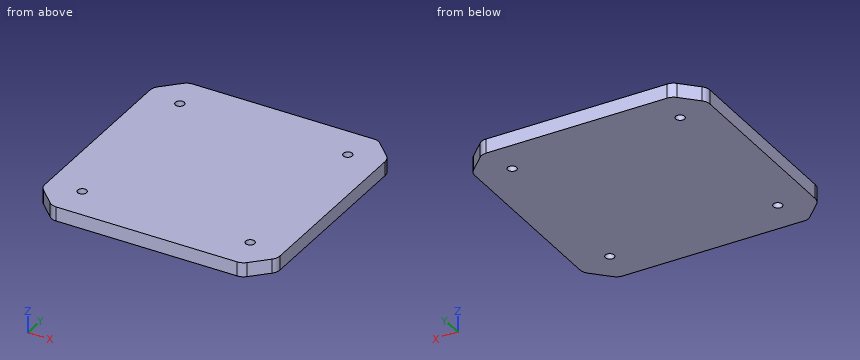
from build123d import *

# Parameters (mm, degrees)
F0_W     = 105
F0_H     = 105
F0_R     = 2
F1_DEPTH = 6.35
F2_SIZE  = 10
F3_R     = 5


# Not quite as in the source:
# - a length typed as a fraction of an inch, garbled in the dataset ("3 / 203.2 mm" for 3/8 in), is restored


with BuildPart() as f1:
    # F0 (on Top) → F1 (new body)
    with BuildSketch(Plane.XY):
        Rectangle(F0_W, F0_H)
        with Locations((-37.5, -37.5)):
            Circle(F0_R, mode=Mode.SUBTRACT)
        with Locations((37.5, -37.5)):
            Circle(F0_R, mode=Mode.SUBTRACT)
        with Locations((-37.5, 37.5)):
            Circle(F0_R, mode=Mode.SUBTRACT)
        with Locations((37.5, 37.5)):
            Circle(F0_R, mode=Mode.SUBTRACT)
    extrude(amount=F1_DEPTH)

    # F2
    f2_edges = [f1.edges().sort_by_distance(p)[0] for p in [
        (-52.5, -52.5, 3.175),
        (52.5, -52.5, 3.175),
        (52.5, 52.5, 3.175),
        (-52.5, 52.5, 3.175),
    ]]
    chamfer(f2_edges, length=F2_SIZE)

    # F3
    f3_edges = [f1.edges().sort_by_distance(p)[0] for p in [
        (52.5, 42.5, 3.175),
        (42.5, 52.5, 3.175),
        (-42.5, 52.5, 3.175),
        (-52.5, 42.5, 3.175),
        (-52.5, -42.5, 3.175),
        (-42.5, -52.5, 3.175),
        (42.5, -52.5, 3.175),
        (52.5, -42.5, 3.175),
    ]]
    fillet(f3_edges, radius=F3_R)


solid = f1.part
Input: part model. Units: mm. Frame: model coordinates. Coordinates: 2 decimals unless noted, no trailing zeros. Order: outer loops, then holes, each group sorted by start corner. A loop starts at its lowest first (then second) coordinate and runs counter-clockwise, first axis right, second up. Notation, with made-up numbers: M 65.25,-26 L 106.25,-26 A14 cw 106.25,-4 Z; hole C 84.5,58 d6. An arc over 180 degrees is marked long. One line per question, with ' | ' between items.
Item 1: Section A-A (z = 1). Output: boundary loops of the cut face in (x, y), then the cut area to 3 significant figures.
Geometry results:
outline: M -52.5,-40.43 A5 ccw -51.04,-43.96 L -43.96,-51.04 A5 ccw -40.43,-52.5 L 40.43,-52.5 A5 ccw 43.96,-51.04 L 51.04,-43.96 A5 ccw 52.5,-40.43 L 52.5,40.43 A5 ccw 51.04,43.96 L 43.96,51.04 A5 ccw 40.43,52.5 L -40.43,52.5 A5 ccw -43.96,51.04 L -51.04,43.96 A5 ccw -52.5,40.43 Z; hole C -37.5,-37.5 d4; hole C -37.5,37.5 d4; hole C 37.5,-37.5 d4; hole C 37.5,37.5 d4 | area: 10,800 mm^2
Item 2: Pin query (flat end, axial travel): pin 1 (2.5 mm diameter, centred on x = 37.5, y = 37.5, fed in from +Z). Return the tip coordinate at first contact, or that it passes through.
Geometry results:
pin 1: passes through
Item 3: Ray query, line 1 along Y through (x, z) = (37.5, 4.5); line 2 along X through (y, z) = (44.5, 5.75); line 3 along X through (y, z) = (42, 4.25). Return the intervals inside material, ascending.
Geometry results:
line 1: y = -52.5 to -39.5, -35.5 to 35.5, 39.5 to 52.5 | line 2: x = -50.5 to 50.5 | line 3: x = -52.25 to 52.25
Item 4: Section B-B (y = 37.5). Output: boundary loops of the cut face in (x, z), then the cut area to 3 significant figures.
Geometry results:
outline: M -52.5,0 L -39.5,0 L -39.5,6.35 L -52.5,6.35 Z; M -35.5,0 L 35.5,0 L 35.5,6.35 L -35.5,6.35 Z; M 39.5,0 L 52.5,0 L 52.5,6.35 L 39.5,6.35 Z | area: 616 mm^2
